CAD build for the part. Positions are in the model's coordinates, mm. Give positions to 0.01 mm unless a question says otherwise; leave off trailing zeros. Write each loop counter-clockwise with the first axis right and the second up, starting at its lowest first coordinate (ties: lowest second). Pieces come first, ordered by that corner, then holes. Notation, with made-up numbers: M 76.5,82.25 L 131.5,82.25 A27 ccw 131.5,119.25 Z; hole C 5,40 d1. An arc over 180 degrees is marked long. One line per question, with ' | ' between items. Start each with the question number.
1. Pull direction Z, two halves, no side cores. Call faces 1 (the face through (0, -5, 0)), 2 (the face through (1.972, -9.732, -1.623)), 3 (the face through (2.03, 11.41, -3.71)): released by +Z, released by -Z, zero draft, split by the parting line, or undercut.
2. Flat gauge pins, fed straight in: pin 1 (2 mm diameter, centred on x = 3.5, z = 1, fed in from +Y); pin 2 (2 mm diameter, centred on x = 2.5, z = 7, fed in from -Y); pin 3 (1.2 mm diameter, centred on x = 1.5, y = 1, fed in from +Z). Where does each tip first touch, or does it go through?
3. Cut at B-B, the plane z = 0.25. Write the cut outline in (x, y).
4. Cut at A-A, the plane y = 0. Write the cut outline in (x, z), then the cut area to 3 significant figures.
5. Cut at D-D, the plane z = -5. Write the cut outline in (x, y), then the cut area to 3 significant figures.
6. Wall check: L1, parallel to Z at x = 0.65, y = 6; L2, parallel to Y at x = 1.95, z = 1; L3, parallel to Y at x = 1.95, z = -8.5. Give the ranges that are in metal, low to high.
7. Cut at C-C, the plane y = -4.5. Write the cut outline in (x, z), then the cut area to 3 significant figures.
```python
from build123d import *

# Parameters (mm, degrees)
BASPROSKE_W         = 4
BASPROSKE_H         = 12
TOOTHCUT_DEPTH      = 18.435595774
TEETHCUTS_COUNT     = 10
TEETHCUTS_ANGLE     = 324
BORSKE_R            = 1
BORE_DEPTH          = 50.0000508
SKETCH_1_W          = 8
SKETCH_1_H          = 8
CUT_EXTRUDE_2_DEPTH = 18.131831434


with BuildPart() as part:
    # BasProSke → Base-Revolve (revolve)
    with BuildSketch(Plane(origin=(0, 0, 0), x_dir=(1, 0, 0), z_dir=(0, 1, 0)), mode=Mode.PRIVATE) as base_revolve_sk:
        with Locations((2, 6)):
            Rectangle(BASPROSKE_W, BASPROSKE_H)
    revolve(base_revolve_sk.sketch.rotate(Axis((-10, 0, 0), (1, 0, 0)), 180), axis=Axis((-10, 0, 0), (1, 0, 0)))

    # TooCutSke → ToothCut (cut, through all)
    with BuildSketch(Plane(origin=(0, 0, 0), x_dir=(0, 0, -1), z_dir=(1, 0, 0))):
        with BuildLine():
            ThreePointArc((1.349961767, 7.376489967), (0, 7.499), (-1.349961767, 7.376489967))
            ThreePointArc((-1.349961767, 7.376489967), (-1.644412889, 9.779161882), (-3.270793922, 11.572041837))
            ThreePointArc((-3.270793922, 11.572041837), (0, 12.0254), (3.270793922, 11.572041837))
            ThreePointArc((3.270793922, 11.572041837), (1.644412889, 9.779161882), (1.349961767, 7.376489967))
        make_face()
    toothcut = extrude(amount=TOOTHCUT_DEPTH, mode=Mode.SUBTRACT)

    # TeethCuts: ToothCut ×10 about axis
    teethcuts_axis = Axis((-10, 0, 0), (1, 0, 0))
    for i in range(1, TEETHCUTS_COUNT):
        add(toothcut.rotate(teethcuts_axis, i * TEETHCUTS_ANGLE / (TEETHCUTS_COUNT - 1)), mode=Mode.SUBTRACT)

    # BorSke → Bore (cut, symmetric)
    with BuildSketch(Plane(origin=(0, 0, 0), x_dir=(0, 0, -1), z_dir=(1, 0, 0))):
        with Locations(Location((0, 0, 0), (0, 0, 180))):
            Circle(BORSKE_R)
    extrude(amount=BORE_DEPTH, both=True, mode=Mode.SUBTRACT)

    # Sketch 1 → Cut-Extrude 2 (cut, through all)
    with BuildSketch(Plane.ZY):
        Rectangle(SKETCH_1_W, SKETCH_1_H)
    extrude(amount=-CUT_EXTRUDE_2_DEPTH, mode=Mode.SUBTRACT)


solid = part.part
```
Here are the results:
1) face 1: zero draft | face 2: undercut | face 3: released by -Z
2) pin 1: y = 10.4 | pin 2: y = -7.32 | pin 3: z = 11.99
3) outline: M 0,-7.49 L 4,-7.49 L 4,-4 L 0,-4 Z; M 0,4 L 4,4 L 4,7.49 L 0,7.49 Z
4) outline: M 0,-12 L 4,-12 L 4,-4 L 0,-4 Z; M 0,4 L 4,4 L 4,12 L 0,12 Z | area: 64.0 mm^2
5) outline: M 0,-5.59 L 4,-5.59 L 4,5.59 L 0,5.59 Z | area: 44.7 mm^2
6) L1: -9.78 to -5.95, -4.5 to 4.5, 5.95 to 9.78 | L2: -7.43 to -4, 4 to 7.43 | L3: -7.42 to -4.34, -1.39 to 1.39, 4.34 to 7.42
7) outline: M 0,-8.7 L 4,-8.7 L 4,8.7 L 0,8.7 Z | area: 69.6 mm^2
